```python
from build123d import *

# Parameters (mm, degrees)
BLANKSKE_W          = 60
BLANKSKE_H          = 3.8
BLANK_DEPTH         = 8
TOOTHCUTSIM_DEPTH   = 61.65014427
TEETHCUTS_COUNT     = 25
TEETHCUTS_PITCH     = 2.51327412
EXTRUDE_1_DEPTH     = 8
SKETCH_2_W          = 10
SKETCH_2_H          = 6.666959913
CUT_EXTRUDE_1_DEPTH = 8


with BuildPart() as part:
    # BlankSke → Blank (new body)
    with BuildSketch(Plane.XY):
        with Locations((30, 1.9)):
            Rectangle(BLANKSKE_W, BLANKSKE_H)
    extrude(amount=-BLANK_DEPTH)

    # TooCutSkeSim → ToothCutSim (cut, through all)
    with BuildSketch(Plane.XY):
        Polygon((0.354348296, 2), (-0.354348296, 2), (-1.018739561, 3.8254), (1.018739561, 3.8254), align=None)
    toothcutsim = extrude(amount=-TOOTHCUTSIM_DEPTH, mode=Mode.SUBTRACT)

    # TeethCuts: ToothCutSim ×25
    with Locations(*[(i * TEETHCUTS_PITCH, 0, 0) for i in range(1, TEETHCUTS_COUNT)]):
        add(toothcutsim, mode=Mode.SUBTRACT)

    # 草图1 → 凸台-拉伸1 (add)
    with BuildSketch(Plane.XY):
        with BuildLine():
            Line((60, 0), (65.623907225, 0))
            Line((65.623907225, 0), (69.923907225, 4.183835629))
            Line((69.923907225, 4.183835629), (69.923907225, 7.183835629))
            Line((69.923907225, 7.183835629), (65.923907225, 7.183835629))
            ThreePointArc((65.923907225, 7.183835629), (63.930879619, 3.484662843), (60, 2))
            Line((60, 2), (60, 0))
        make_face()
    extrude(amount=-EXTRUDE_1_DEPTH)

    # 草图2 → 切除-拉伸1 (cut)
    with BuildSketch(Plane.XY):
        with Locations((5, 3.333479957)):
            Rectangle(SKETCH_2_W, SKETCH_2_H)
    extrude(amount=-CUT_EXTRUDE_1_DEPTH, mode=Mode.SUBTRACT)


solid = part.part
```
Geometry check sheet. Reference: the model listing, model coordinates, mm. Coordinates: 2 decimals unless noted, no trailing zeros. Write each loop counter-clockwise with the first axis right and the second up, starting at its lowest first coordinate (ties: lowest second). Pieces come first, ordered by that corner, then holes. Notation, with made-up numbers: M 48,68.5 L 77,68.5 A18 ccw 77,101.5 Z; hole C 60,56 d6. An arc over 180 degrees is marked long. Answer as a JSON object with one key per item and string values.
1. Section check C-C, the plane y = 5.5. Enter the section's corners in (x, z).
Answers below:
{"outline": "M 65.43,-8 L 69.92,-8 L 69.92,0 L 65.43,0 Z"}
2. Draft check along X on faces 1 (the flat face through (28.33, 2.91, -3.94)), 2 (the flat face through (37, 0, -4)), 3 (the flat face through (69.924, 6, -4)). Enter one of: released by +X, released by -X, zero draft, split by the parting line, or undercut.
Answers below:
{"face 1": "undercut", "face 2": "zero draft", "face 3": "released by +X"}
3. Scan lines: L1, parallel to Y at x = 45.5, z = -3; L2, parallel to X at y = 6, z = -4.25; L3, parallel to Y at x = 34, z = -4.75. Record each from-to range of solid material in increasing order.
Answers below:
{"L1": "y = 0 to 2", "L2": "x = 65.64 to 69.92", "L3": "y = 0 to 3.8"}
4. Section check B-B, the plane x = 63.5. Enter the section's corners in (y, z), plus the area to 3 significant figures.
Answers below:
{"outline": "M 0,-8 L 3.14,-8 L 3.14,0 L 0,0 Z", "area": "25.1 mm²"}
5. Go/stop test with flat-tipped pins: pin 1 Ø1 at (x, z) = (22, -2.5) entering from +Y; pin 2 Ø1.5 at (y, z) = (5.5, -1.5) entering from -X; pin 3 Ø2 at (x, y) = (47.5, 5.5) entering from +Z. Record where each tip stops, or that it passes through.
Answers below:
{"pin 1": "stops at y = 3.8", "pin 2": "stops at x = 65.02", "pin 3": "passes through"}
6. Section check A-A, the plane y = 3. Give the number of separate pieces and of enclosed holes in the cut face, plus the area to 3 significant figures.
Answers below:
{"separate pieces": "21", "enclosed holes": "0", "area": "216 mm²"}
